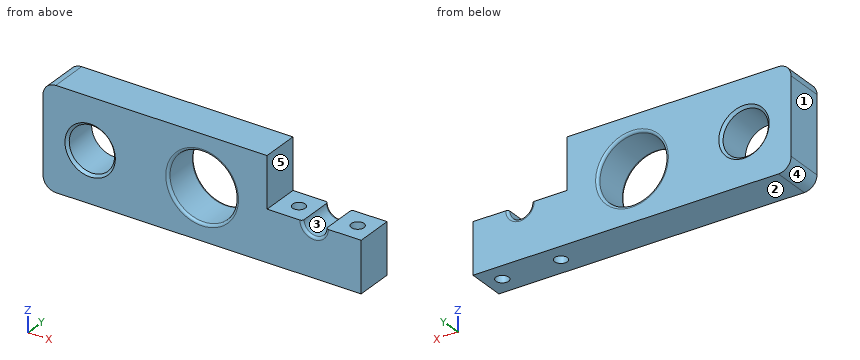
from build123d import *

# Parameters (mm, degrees)
SKETCH_1_W          = 125
SKETCH_1_H          = 40
EXTRUDE_1_DEPTH     = 15
SKETCH_2_R          = 8.9
SKETCH_2_R_2        = 4.6
SKETCH_2_R_3        = 13.3
CUT_EXTRUDE_1_DEPTH = 133.098448136
CHAMFER_1_SIZE      = 1
CHAMFER_2_SIZE      = 1
FILLET_1_R          = 1
SKETCH_5_W          = 40
SKETCH_5_H          = 20
CUT_EXTRUDE_2_DEPTH = 133.098448148
FILLET_4_R          = 5
SKETCH_12_W         = 3.06
SKETCH_12_H         = 20
EXTRUDE_2_DEPTH     = 15
SKETCH_14_R         = 2.5
CUT_EXTRUDE_3_DEPTH = 128.47548784


with BuildPart() as part:
    # 草圖1 → 填料-伸長1 (new body)
    with BuildSketch(Plane(origin=(0, 0, 0), x_dir=(1, 0, 0), z_dir=(0, 1, 0))):
        with Locations((62.5, 20)):
            Rectangle(SKETCH_1_W, SKETCH_1_H)
    extrude(amount=EXTRUDE_1_DEPTH)

    # 草圖2 → 除料-伸長1 (cut, through all)
    with BuildSketch(Plane(origin=(0, 15, 0), x_dir=(1, 0, 0), z_dir=(0, 1, 0))):
        with Locations(Location((18.526668527, 20, 0), (0, 0, 270))):
            Circle(SKETCH_2_R)
        with Locations(Location((106.526668527, 20, 0), (0, 0, 270))):
            Circle(SKETCH_2_R_2)
        with Locations(Location((62.526668527, 20, 0), (0, 0, 270))):
            Circle(SKETCH_2_R_3)
    extrude(amount=-CUT_EXTRUDE_1_DEPTH, mode=Mode.SUBTRACT)

    # 導角1
    chamfer_1_edges = [part.edges().sort_by_distance(p)[0] for p in [
        (18.526668527, 15, -28.9),
    ]]
    chamfer(chamfer_1_edges, length=CHAMFER_1_SIZE)

    # 導角2
    chamfer_2_edges = [part.edges().sort_by_distance(p)[0] for p in [
        (18.526668527, 0, -28.9),
    ]]
    chamfer(chamfer_2_edges, length=CHAMFER_2_SIZE)

    # 圓角1
    fillet_1_edges = [part.edges().sort_by_distance(p)[0] for p in [
        (106.526668527, 0, -24.6),
        (106.526668527, 15, -24.6),
        (62.526668527, 0, -33.3),
        (62.526668527, 15, -33.3),
    ]]
    fillet(fillet_1_edges, radius=FILLET_1_R)

    # 草圖5 → 除料-伸長2 (cut, through all)
    with BuildSketch(Plane(origin=(0, 15, 0), x_dir=(1, 0, 0), z_dir=(0, 1, 0))):
        with Locations((105, 10)):
            Rectangle(SKETCH_5_W, SKETCH_5_H)
    extrude(amount=-CUT_EXTRUDE_2_DEPTH, mode=Mode.SUBTRACT)

    # 圓角4
    fillet_4_edges = [part.edges().sort_by_distance(p)[0] for p in [
        (0, 7.5, -40),
        (0, 7.5, 0),
    ]]
    fillet(fillet_4_edges, radius=FILLET_4_R)

    # 草圖12 → 填料-伸長2 (add)
    with BuildSketch(Plane(origin=(0, 15, 0), x_dir=(1, 0, 0), z_dir=(0, 1, 0))):
        with Locations((86.53, 10)):
            Rectangle(SKETCH_12_W, SKETCH_12_H)
    extrude(amount=-EXTRUDE_2_DEPTH)

    # 草圖14 → 除料-伸長3 (cut, through all)
    with BuildSketch(Plane.XY.offset(-20)):
        with Locations((118.565, 7.5)):
            Circle(SKETCH_14_R)
        with Locations((95.491668527, 7.5)):
            Circle(SKETCH_14_R)
    extrude(amount=-CUT_EXTRUDE_3_DEPTH, mode=Mode.SUBTRACT)


solid = part.part
Model file for the job. Use its own axes, mm. Face numbers are marked on the shaded views. A direction names the side the tool comes from. Round coordinates to 2 decimals unless told otherwise and drop trailing zeros. Order: outer loops, then holes, each group sorted by start corner. A loop starts at its lowest first (then second) coordinate and runs counter-clockwise, first axis right, second up.
(1) Band-saw the part on A-A (y = 7.5). List the corners of the cut face in (x, z) (3 decimals).
(2) Band-saw the part on B-B (z = -27). Give the number of separate pieces and of enclosed holes in the cut face, then the cut area to 3 significant figures.
(3) 3-axis set-ups, long thin cutter, end or side, ignore diameter. For the marked faces 4 and 5: which of +Z, -Z, +X, -X, +Y, -Y reach the whole face in a straight line?
(4) Pull direction X, two halves, no side cores. Call the marked faces 1, 2 and 3: released by +X, released by -X, zero draft, split by the parting line, or undercut.
(5) Pin check, flat tips, straight feed: pin 1 (4 mm diameter, centred on x = 97.5, y = 8.5, fed in from +Z); pin 2 (4.5 mm diameter, centred on y = 4, z = -11.5, fed in from +X). Stop position of each tip, or through.
(6) Drill centre lines: line 1 (X direction, y = 13.5, z = -22); line 2 (X direction, y = 3.75, z = -16.5); line 3 (X direction, y = 1, z = -20.5). Where is each one in solid material? Low to high.
Verdict:
1. outline: (0, -35) arc R5 ccw to (5, -40) - (92.992, -40) - (92.992, -20) - (88.06, -20) - (88.06, 0) - (5, 0) arc R5 ccw to (0, -5) - close; (97.992, -40) - (116.065, -40) - (116.065, -20) - (111.127, -20) arc R4.6 cw to (101.927, -20) - (97.992, -20) - close; (121.065, -40) - (125, -40) - (125, -20) - (121.065, -20) - close; hole circle Ø17.8 at (18.527, -20); hole circle Ø26.6 at (62.527, -20)
2. separate pieces: 3
2. enclosed holes: 2
2. area: 1,330 mm2
3. face 4: -Z, -X, +Y, -Y
3. face 5: +Z, +X, +Y, -Y
4. face 1: released by -X
4. face 2: zero draft
4. face 3: undercut
5. pin 1: stops at z = -20
5. pin 2: stops at x = 88.06
6. line 1: x = 0 to 9.85, 27.2 to 49.38, 75.68 to 102.38, 110.67 to 125
6. line 2: x = 0 to 10.34, 26.71 to 49.7, 75.36 to 88.06
6. line 3: x = 0 to 9.64, 27.41 to 49.24, 75.82 to 101.95, 111.1 to 125
